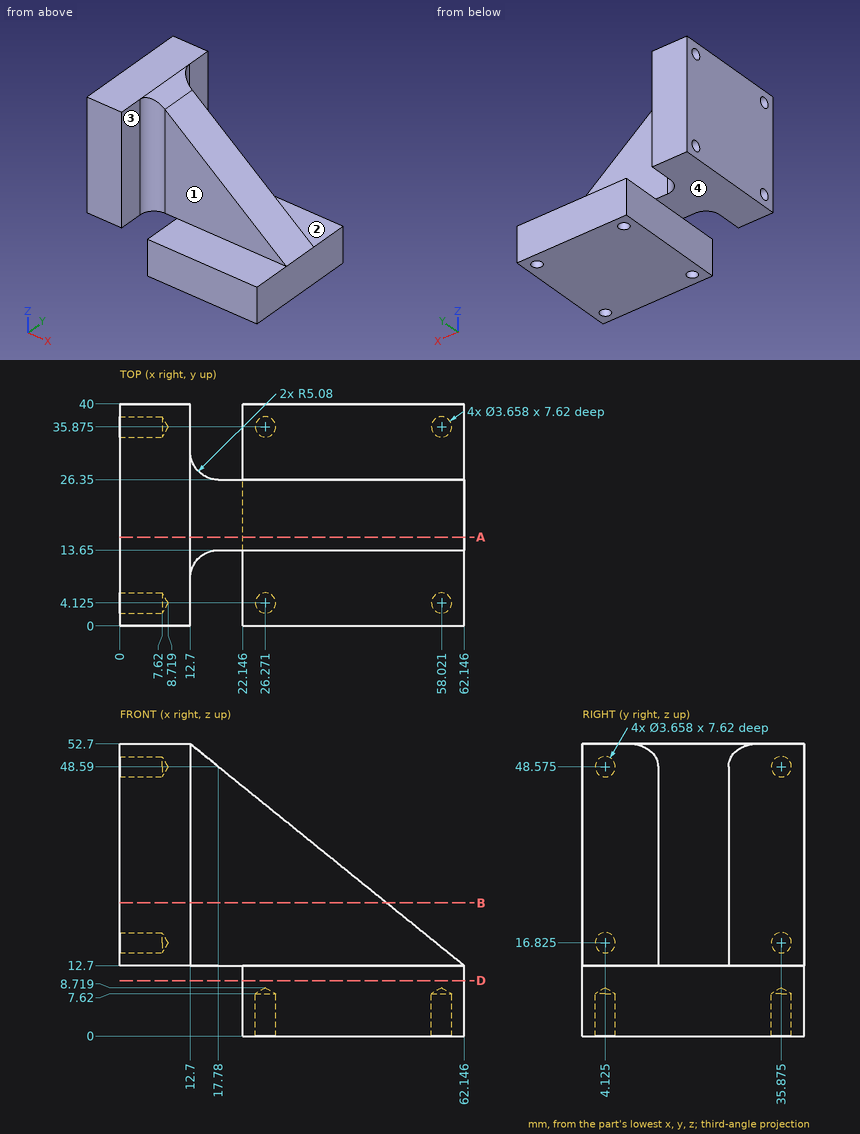
Answer from the drawing. Dimensions are ordinates in mm from the lowest x, y and z of the part. A direction names the side the tool comes from. Coordinates: 2 decimals unless noted, no trailing zeros. Write each loop counter-clockwise with the first axis right and the second up, starting at its lowest first coordinate (ties: lowest second). Pieces come first, ordered by that corner, then holes. Notation, with made-up numbers: M 5.5,86 L 39.5,86 A21 cw 39.5,92 Z; hole C 73,84.5 d9. An arc over 180 degrees is marked long. Use a Markdown table: item, result.
Q1. Straight lines are drawn through the part: L1, parallel to Z at x = 3, y = 32.5; L2, parallel to X at y = 9, z = 13; L3, parallel to Z at x = 36.5, y = 34. For each, find the intervals that lie inside material, in ascending order. Write a range as [from, to].
Answer block:
| item | result |
|---|---|
| L1 | z = [12.7, 52.7] |
| L2 | x = [0, 12.72] |
| L3 | z = [0, 12.7] |
Q2. The part is cut by section B-B, the plane z = 24. Write down the section's boundary in (x, y).
Answer block:
| item | result |
|---|---|
| outline | M 0,0 L 12.7,0 L 12.7,8.57 A5.08 cw 17.78,13.65 L 48.18,13.65 L 48.18,26.35 L 17.78,26.35 A5.08 cw 12.7,31.43 L 12.7,40 L 0,40 Z |
Q3. The part is cut by section A-A, the plane y = 16. Write down the section's boundary in (x, z).
Answer block:
| item | result |
|---|---|
| outline | M 0,12.7 L 22.15,12.7 L 22.15,0 L 62.15,0 L 62.15,12.7 L 12.7,52.7 L 0,52.7 Z |
Q4. Each of these flat-tipped pins is pushed along its axis until it touches: pin 1 Ø3 at (y, z) = (4.12, 48.57) entering from +X; pin 2 Ø11 at (x, z) = (29.5, 31) entering from +Y; pin 3 Ø4 at (y, z) = (27.5, 5.5) entering from -X. Where does it stop, or does it pass through?
Answer block:
| item | result |
|---|---|
| pin 1 | stops at x = 12.7 |
| pin 2 | stops at y = 26.35 |
| pin 3 | stops at x = 22.15 |
Q5. The part is cut by section D-D, the plane z = 10. Write down the section's boundary in (x, y), then the cut area to 3 significant figures.
Answer block:
| item | result |
|---|---|
| outline | M 22.15,0 L 62.15,0 L 62.15,40 L 22.15,40 Z |
| area | 1,600 mm2 |
Q6. Which of the six approach directions +Z, -Z, +X, -X, +Y, -Y give full straight-line access (tool end or side, diameter ignored) to the marked faces 1, 2, 3 and 4?
Answer block:
| item | result |
|---|---|
| face 1 | +Z, +X, -Y |
| face 2 | +Z, +X, +Y |
| face 3 | +Z, -Z, +X, -Y |
| face 4 | -Z, -X, +Y, -Y |
